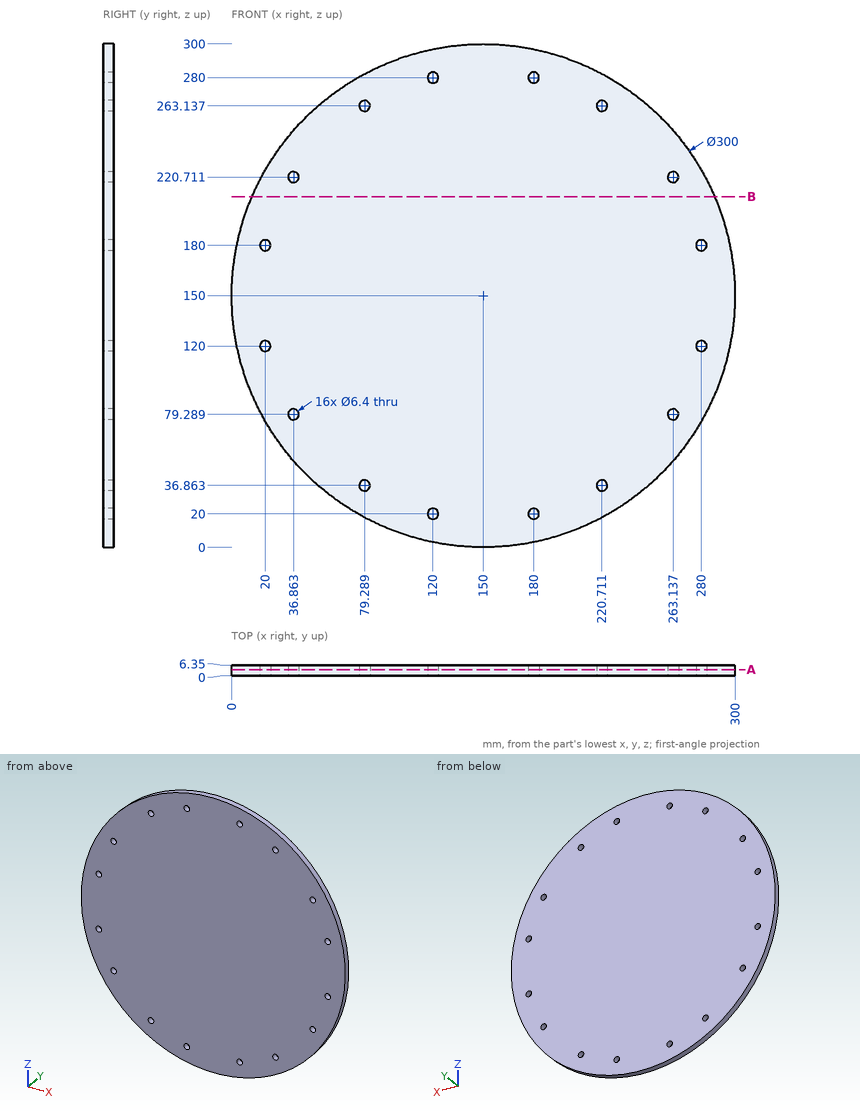
The drawing under review shows one solid part. Ordinate dimensions are in mm from its lowest x, y, z. Coordinates: 2 decimals unless noted, no trailing zeros. Order: outer loops, then holes, each group sorted by start corner. A loop starts at its lowest first (then second) coordinate and runs counter-clockwise, first axis right, second up. Notation, with made-up numbers: (63.25, 28) -> (86.25, 28) arc R14 cw to (86.25, 41) -> close; hole circle Ø10 at (4, -12.75). An arc over 180 degrees is marked (long way). Use CSV: the item, a comma, the result in double quotes. Start each with the question number.
Item 1: We need section B-B, the plane z = 209. Give the boundary of the cut face in (x, y), then the cut area to 3 significant figures.
Item 2: Insertion check: pin 1 (3 mm diameter, centred on x = 206, y = 3.5, fed in from +Z); pin 2 (1.5 mm diameter, centred on y = 2.5, z = 176, fed in from -X); pin 3 (1.5 mm diameter, centred on y = 2.5, z = 208.5, fed in from -X). Each pin has a flat end and moves straight along its axis. Give the tip position at first contact, or say it passes through.
Item 3: We need section A-A, the plane y = 3.75. Give the number of separate pieces and of enclosed holes in the cut face, then the cut area to 3 significant figures.
Item 4: Wall thickness on probe 1 along X at (y, z) = (1.25, 37) (1 decimal); probe 2 along Z at (x, y) = (20, 4) (1 decimal); probe 3 along X at (y, z) = (0.75, 146): over which ranges is each line inside the solid? List them lowest first.
Derived:
1,outline,"(12.09, 0) -> (287.91, 0) -> (287.91, 6.35) -> (12.09, 6.35) -> close"
1,area,"1,750 mm^2"
2,pin 1,"stops at z = 289.75"
2,pin 2,"stops at x = 2.14"
2,pin 3,"stops at x = 11.56"
3,separate pieces,"1"
3,enclosed holes,"16"
3,area,"70,200 mm^2"
4,probe 1,"x = 51.4 to 76.1, 82.5 to 217.5, 223.9 to 248.6"
4,probe 2,"z = 75.2 to 116.8, 123.2 to 176.8, 183.2 to 224.8"
4,probe 3,"x = 0.05 to 299.95"
